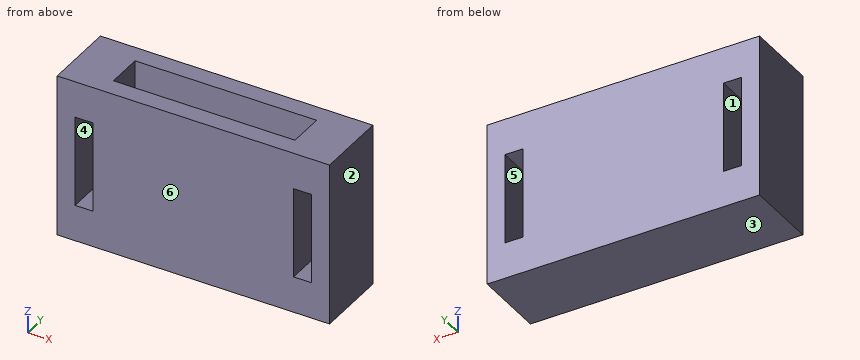
```python
from build123d import *

# Parameters (mm, degrees)
SKETCH1_W           = 38.1
SKETCH1_H           = 22.86
SKETCH1_W_2         = 2.54
SKETCH1_H_2         = 12.7
BOSS_EXTRUDE2_DEPTH = 2.54
SKETCH3_R           = 1.016
BOSS_EXTRUDE3_DEPTH = 5.08
BOSS_EXTRUDE5_DEPTH = 5.08
SKETCH6_W           = 2.54
SKETCH6_H           = 12.7
CUT_EXTRUDE1_DEPTH  = 24.486417351
SKETCH4_W           = 38.1
SKETCH4_H           = 22.86
SKETCH4_W_2         = 2.54
SKETCH4_H_2         = 12.7
BOSS_EXTRUDE6_DEPTH = 2.54


with BuildPart() as part:
    # Sketch1 → Boss-Extrude2 (new body)
    with BuildSketch(Plane(origin=(0, 0, 0), x_dir=(1, 0, 0), z_dir=(0, 1, 0))):
        Rectangle(SKETCH1_W, SKETCH1_H)
        with Locations((-15.28489899, 0)):
            Rectangle(SKETCH1_W_2, SKETCH1_H_2, mode=Mode.SUBTRACT)
        with Locations((15.28489899, 0)):
            Rectangle(SKETCH1_W_2, SKETCH1_H_2, mode=Mode.SUBTRACT)
    extrude(amount=BOSS_EXTRUDE2_DEPTH)

    # Sketch3 → Boss-Extrude3 (add)
    with BuildSketch(Plane(origin=(0, 2.54, 0), x_dir=(1, 0, 0), z_dir=(0, 1, 0))):
        with Locations(Location((-5.318941048, 2.54, 0), (0, 0, 90))):
            Circle(SKETCH3_R)
        with Locations(Location((5.318941048, 2.54, 0), (0, 0, 90))):
            Circle(SKETCH3_R)
    extrude(amount=BOSS_EXTRUDE3_DEPTH)

    # Sketch5 → Boss-Extrude5 (add)
    with BuildSketch(Plane(origin=(0, 2.54, 0), x_dir=(1, 0, 0), z_dir=(0, 1, 0))):
        Polygon((-19.05, -11.43), (-19.05, 11.43), (19.05, 11.43), (19.05, -11.43), (12.7, -11.43), (12.7, 6.35), (-12.7, 6.35), (-12.7, -11.43), align=None)
    extrude(amount=BOSS_EXTRUDE5_DEPTH)

    # Sketch6 → Cut-Extrude1 (cut, through all)
    with BuildSketch(Plane(origin=(0, 7.62, 0), x_dir=(1, 0, 0), z_dir=(0, 1, 0))):
        with Locations((-15.28489899, 0)):
            Rectangle(SKETCH6_W, SKETCH6_H)
        with Locations((15.28489899, 0)):
            Rectangle(SKETCH6_W, SKETCH6_H)
    extrude(amount=-CUT_EXTRUDE1_DEPTH, mode=Mode.SUBTRACT)

    # Sketch4 → Boss-Extrude6 (add)
    with BuildSketch(Plane(origin=(0, 7.62, 0), x_dir=(1, 0, 0), z_dir=(0, 1, 0))):
        Rectangle(SKETCH4_W, SKETCH4_H)
        with Locations((-15.28489899, 0)):
            Rectangle(SKETCH4_W_2, SKETCH4_H_2, mode=Mode.SUBTRACT)
        with Locations((15.28489899, 0)):
            Rectangle(SKETCH4_W_2, SKETCH4_H_2, mode=Mode.SUBTRACT)
    extrude(amount=BOSS_EXTRUDE6_DEPTH)


solid = part.part
```
Here's how the part is built. I have some questions about the finished solid (model axes, mm). Face numbers are marked on the shaded views. A direction names the side the tool comes from. Give positions to 0.01 mm unless a question says otherwise; leave off trailing zeros. Loops run counter-clockwise (first coordinate to the right, second up) from the corner with the lowest first, then second, coordinate; pieces in that order, holes last. Notation, with made-up numbers: M -27,-25.5 L 18,-25.5 A30 ccw 18,-2.5 Z; hole C 49.25,86 d8. An arc over 180 degrees is marked long. Put each result on its own line as item: value. Start each with the question number.
(1) I want a section at C-C on z = -2.54. Please give me the cut outline in (x, y), then the cut area to 3 significant figures.
(2) I need wall thicknesses on line 1 along X through (y, z) = (4.5, -4.75); line 2 along X through (y, z) = (9.5, -6); line 3 along Y through (x, z) = (12, 4.75). Which ranges of each line are inside material? Lowest first, please. Write a range as [from, to].
(3) If we mould it in two halves opening along Z, with no side actions, what happens to the marked faces 1, 2, 3 and 4? For each: +Z half, -Z half, draft (parallel to the pull), parting line (faces both ways), or undercut.
(4) I want a section at B-B on y = 1.5. Please give me the cut outline in (x, z), then the cut area to 3 significant figures.
(5) I want a section at A-A on z = 2.5. Please give me the cut outline in (x, y).
(6) Will this pin go through, and if not, where does the flat tip stop? pin 1 Ø1.5 at (x, y) = (-1.5, 4) entering from +Z.
(7) For the marked faces 5 and 6, which set-ups out of +Z, -Z, +X, -X, +Y, -Y let a thin tool reach every point of the face, with its end or its side?
(8) I want a section at D-D on x = -7.5. Please give me the cut outline in (y, z), then the cut area to 3 significant figures.
Answer block:
1. outline: M -19.05,0 L -16.55,0 L -16.55,10.16 L -19.05,10.16 Z; M -14.01,0 L 14.01,0 L 14.01,10.16 L -14.01,10.16 Z; M 16.55,0 L 19.05,0 L 19.05,10.16 L 16.55,10.16 Z; hole M -12.7,2.54 L -6.33,2.54 L -6.33,7.62 L -12.7,7.62 Z; hole M -4.3,2.54 L 4.3,2.54 L 4.3,7.62 L -4.3,7.62 Z; hole M 6.33,2.54 L 12.7,2.54 L 12.7,7.62 L 6.33,7.62 Z
1. area: 227 mm^2
2. line 1: [-19.05, -16.55], [-14.01, -12.7], [12.7, 14.01], [16.55, 19.05]
2. line 2: [-19.05, -16.55], [-14.01, 14.01], [16.55, 19.05]
2. line 3: [0, 2.54], [7.62, 10.16]
3. face 1: undercut
3. face 2: draft
3. face 3: -Z half
3. face 4: undercut
4. outline: M -19.05,-11.43 L 19.05,-11.43 L 19.05,11.43 L -19.05,11.43 Z; hole M -16.55,-6.35 L -14.01,-6.35 L -14.01,6.35 L -16.55,6.35 Z; hole M 14.01,-6.35 L 16.55,-6.35 L 16.55,6.35 L 14.01,6.35 Z
4. area: 806 mm^2
5. outline: M -19.05,0 L -16.55,0 L -16.55,10.16 L -19.05,10.16 Z; M -14.01,0 L 14.01,0 L 14.01,10.16 L -14.01,10.16 Z; M 16.55,0 L 19.05,0 L 19.05,10.16 L 16.55,10.16 Z; hole M -12.7,2.54 L 12.7,2.54 L 12.7,7.62 L -12.7,7.62 Z
6. pin 1: z = -6.35
7. face 5: +Y, -Y
7. face 6: +Z, -Z, +X, -X, -Y
8. outline: M 0,-11.43 L 10.16,-11.43 L 10.16,11.43 L 7.62,11.43 L 7.62,-6.35 L 2.54,-6.35 L 2.54,11.43 L 0,11.43 Z
8. area: 142 mm^2
